Part model, mm, in its own coordinate system. Face numbers are marked on the shaded views. Round coordinates to 2 decimals unless told otherwise and drop trailing zeros. Loops run counter-clockwise (first coordinate to the right, second up) from the corner with the lowest first, then second, coordinate; pieces in that order, holes last. Notation, with made-up numbers: (39.5, -35.75) - (48.5, -35.75) arc R24 ccw to (48.5, -15.75) - close; hole circle Ø7 at (40, 37.5). An arc over 180 degrees is marked (long way). Write each question's results on one line, items separated by ' | '. Start each with the question number.
(1) Flat gauge pins, fed straight in: P1, Ø1, axis at x = 14, y = -1.5, coming from the -Z side; P2, Ø0.5, axis at y = 0, z = -62.5, coming from the -X side; P3, Ø2.5, axis at x = 7.5, y = -1.5, coming from the +Z side; P4, Ø3, axis at y = 0, z = 0, coming from the +X side. Where does each tip first touch, or does it go through?
(2) Cut at C-C, the plane z = -46.5. List the corners of the cut face in (x, y).
(3) Drill centre lines: L1, parallel to Y at x = 1, z = -106.5; L2, parallel to Y at x = 10.35, z = -117; L3, parallel to Z at x = -14, y = -0.75. Where is each one in solid material? Low to high.
(4) Cut at B-B, the plane z = 0. List the corners of the cut face in (x, y), then the cut area to 3 significant figures.
(5) Cut at A-A, the plane x = 0. Give the number of separate pieces and of enclosed holes in the cut face, then the cut area to 3 significant figures.
(6) Cut at D-D, the plane z = -13. List the corners of the cut face in (x, y), then the cut area to 3 significant figures.
(7) Mould opens along Z. For the marked faces 1, 2 and 3 say: released by +Z, released by -Z, zero draft, split by the parting line, or undercut.
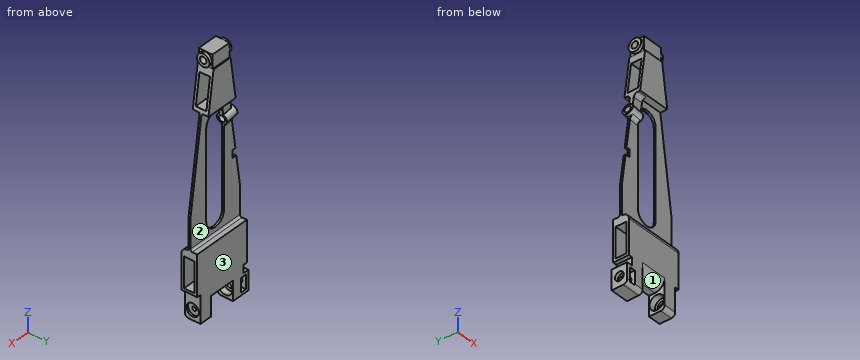
from build123d import *

# Parameters (mm, degrees)
JOINTTIBIA_DEPTH           = 3.5
JOINTTIBIA_DEPTH_BACK      = 3.5
ESQUISSE2_W                = 13.5
ESQUISSE2_H                = 7
ESQUISSE3_R                = 1.7
HOLEAXETIBIA_DEPTH         = 14.5
ESQUISSE4_R                = 5.505678288
ESQUISSE4_R_2              = 3.2
ENTRETOISETIBIA_DEPTH      = 1.5
SHAPEJOINTCOXA_DEPTH       = 4
SHAPEJOINTCOXA_DEPTH_BACK  = 4
ESQUISSE6_R                = 3.2
HOLEMAGNET_DEPTH           = 1
ESQUISSE7_R                = 2.25
HOLEAXE_DEPTH              = 8
ESQUISSE9_R                = 3.7
HOLEBEARING_DEPTH          = 3.2
ESQUISSE10_R               = 2.25
ENTRETOISEBEARING_DEPTH    = 1
ESQUISSE12_W               = 10
ESQUISSE12_H               = 8
ESQUISSE12_R               = 2.25
EXTSCREWLESS_DEPTH         = 3
ESQUISSE13_W               = 3
ESQUISSE13_H               = 7
SCEWLESSLOCKER_DEPTH       = 10
ESQUISSE24_W               = 30.5
ESQUISSE24_H               = 8
SHAPE_BDY_DEPTH            = 104.5
TRIANGULIZE_DEPTH          = 10
ESQUISSE27_W               = 15.4
ESQUISSE27_H               = 5.4
ATTACHWINGS_DEPTH          = 10
ESQUISSE29_W               = 62.63923601
ESQUISSE29_H               = 9.700813627
VOID_BODY_DEPTH            = 38
MASS_REMOVER_PCB_DEPTH     = 10
CONG_1_R                   = 5
CONG_2_R                   = 3
ESQUISSE32_W               = 15.4
ESQUISSE32_H               = 5.4
LOCKERHOLE_DEPTH           = 32
FIXATIONSENSOR_DEPTH       = 1.5
FIXATIONSENSOR_DEPTH_BACK  = 5
ESQUISSE33_R               = 2.6
ESQUISSE34_R               = 1.6
SCREWFIXATIONSENSOR_DEPTH  = 10
ESQUISSE35_W               = 8
ESQUISSE35_H               = 2
FIXATIONSENSORRENFOR_DEPTH = 5
CONG_3_R                   = 3
CONG_4_R                   = 2
CONG_5_R                   = 2
CONG_6_R                   = 1
ESQUISSE36_R               = 2
ENL_V_MAT_EXTRU_1_DEPTH    = 4.5
ESQUISSE38_R               = 1
REMOVER_HELPER_DEPTH       = 10


with BuildPart() as part:
    # Esquisse2 → JointTibia (new, two sides: drawn at the far end of the back side and taken through both)
    with BuildSketch(Plane(origin=(0, 0, 0), x_dir=(1, 0, 0), z_dir=(0, 1, 0)).offset(-JOINTTIBIA_DEPTH_BACK)):
        Rectangle(ESQUISSE2_W, ESQUISSE2_H)
    extrude(amount=JOINTTIBIA_DEPTH + JOINTTIBIA_DEPTH_BACK)

    # Esquisse3 → HoleAxeTibia (cut)
    with BuildSketch(Plane(origin=(6.75, 0, 0), x_dir=(0, 0, -1), z_dir=(1, 0, 0))):
        Circle(ESQUISSE3_R)
    extrude(amount=-HOLEAXETIBIA_DEPTH, mode=Mode.SUBTRACT)

    # Esquisse4 → EntretoiseTibia (cut)
    with BuildSketch(Plane(origin=(6.75, 0, 0), x_dir=(0, 0, -1), z_dir=(1, 0, 0))):
        Circle(ESQUISSE4_R)
        Circle(ESQUISSE4_R_2, mode=Mode.SUBTRACT)
    entretoisetibia = extrude(amount=-ENTRETOISETIBIA_DEPTH, mode=Mode.SUBTRACT)

    # Symétrie1: EntretoiseTibia across plane
    add(entretoisetibia.mirror(Plane(origin=(0, 0, 0), x_dir=(0, 0, 1), z_dir=(1, 0, 0))), mode=Mode.SUBTRACT)



with BuildPart() as body_2:
    # Esquisse5 → ShapeJointCoxa (new, two sides: drawn at the far end of the back side and taken through both)
    with BuildSketch(Plane(origin=(0, 0, 0), x_dir=(1, 0, 0), z_dir=(0, 1, 0)).offset(-SHAPEJOINTCOXA_DEPTH_BACK)):
        Polygon((-13.25, 112), (-13.25, 122), (-6.75, 122), (-6.75, 112), (6.75, 112), (6.75, 122), (13.25, 122), (13.25, 112), (13.25, 108), (-13.25, 108), align=None)
    extrude(amount=SHAPEJOINTCOXA_DEPTH + SHAPEJOINTCOXA_DEPTH_BACK)

    # Esquisse6 → HoleMagnet (cut)
    with BuildSketch(Plane(origin=(13.25, 0, 0), x_dir=(0, 0, -1), z_dir=(1, 0, 0))):
        with Locations((117, 0)):
            Circle(ESQUISSE6_R)
    extrude(amount=-HOLEMAGNET_DEPTH, mode=Mode.SUBTRACT)

    # Esquisse7 → HoleAxe (cut)
    with BuildSketch(Plane.ZY.offset(13.25)):
        with Locations((-117, 0)):
            Circle(ESQUISSE7_R)
    extrude(amount=-HOLEAXE_DEPTH, mode=Mode.SUBTRACT)

    # Esquisse9 → HoleBearing (cut)
    with BuildSketch(Plane.ZY.offset(-6.75)):
        with Locations((-117, 0)):
            Circle(ESQUISSE9_R)
    holebearing = extrude(amount=-HOLEBEARING_DEPTH, mode=Mode.SUBTRACT)

    # Symétrie2: HoleBearing across plane
    add(holebearing.mirror(Plane(origin=(0, 0, 0), x_dir=(0, 0, 1), z_dir=(1, 0, 0))), mode=Mode.SUBTRACT)

    # Esquisse10 → EntretoiseBearing (cut)
    with BuildSketch(Plane.ZY.offset(-9.95)):
        with Locations((-117, 0)):
            Circle(ESQUISSE10_R)
    extrude(amount=-ENTRETOISEBEARING_DEPTH, mode=Mode.SUBTRACT)

    # Esquisse12 → ExtScrewLess (add)
    with BuildSketch(Plane.ZY.offset(13.25)):
        with Locations((-117, 0)):
            Rectangle(ESQUISSE12_W, ESQUISSE12_H)
        with Locations((-117, 0)):
            Circle(ESQUISSE12_R, mode=Mode.SUBTRACT)
    extrude(amount=EXTSCREWLESS_DEPTH)

    # Esquisse13 → ScewLessLocker (cut)
    with BuildSketch(Plane(origin=(0, 4, 0), x_dir=(1, 0, 0), z_dir=(0, 1, 0))):
        with Locations((-13.1, 117)):
            Rectangle(ESQUISSE13_W, ESQUISSE13_H)
    extrude(amount=-SCEWLESSLOCKER_DEPTH, mode=Mode.SUBTRACT)


with BuildPart() as part_1:
    add(part.part)

    add(body_2.part)  # Shape_bdy merges body 2
    # Esquisse24 → Shape_bdy (add)
    with BuildSketch(Plane.XY.offset(-108)):
        Rectangle(ESQUISSE24_W, ESQUISSE24_H)
    extrude(amount=SHAPE_BDY_DEPTH)

    # Esquisse26 → Triangulize (cut)
    with BuildSketch(Plane.XZ.offset(4)):
        Polygon((-5.25, -3.5), (-15.25, -72), (-15.25, -3.5), align=None)
        Polygon((5.25, -3.5), (15.25, -3.5), (15.25, -72), align=None)
    extrude(amount=-TRIANGULIZE_DEPTH, mode=Mode.SUBTRACT)

    # Esquisse27 → AttachWings (cut)
    with BuildSketch(Plane(origin=(15.25, 0, 0), x_dir=(0, 0, -1), z_dir=(1, 0, 0))):
        with Locations((99, 0)):
            Rectangle(ESQUISSE27_W, ESQUISSE27_H)
        with Locations((15, 0)):
            Rectangle(ESQUISSE27_W, ESQUISSE27_H)
    attachwings = extrude(amount=-ATTACHWINGS_DEPTH, mode=Mode.SUBTRACT)

    # Symétrie4: AttachWings across plane
    add(attachwings.mirror(Plane(origin=(0, 0, 0), x_dir=(0, 0, 1), z_dir=(1, 0, 0))), mode=Mode.SUBTRACT)

    # Esquisse29 → Void body (cut)
    with BuildSketch(Plane(origin=(15.25, 0, 0), x_dir=(0, 0, -1), z_dir=(1, 0, 0))):
        with Locations((56.023105982, 5.350406814)):
            Rectangle(ESQUISSE29_W, ESQUISSE29_H)
        with Locations((56.023105982, -5.350406814)):
            Rectangle(ESQUISSE29_W, ESQUISSE29_H)
    extrude(amount=-VOID_BODY_DEPTH, mode=Mode.SUBTRACT)

    # Esquisse30 → Mass remover & PCB (cut)
    with BuildSketch(Plane(origin=(0, 0.5, 0), x_dir=(1, 0, 0), z_dir=(0, 1, 0))):
        with BuildLine():
            Line((5.5, 78.523105982), (5.5, 33.523105982))
            ThreePointArc((5.5, 33.523105982), (0, 28.023105982), (-5.5, 33.523105982))
            Line((-5.5, 33.523105982), (-5.5, 78.523105982))
            ThreePointArc((-5.5, 78.523105982), (0, 84.023105982), (5.5, 78.523105982))
        make_face()
    extrude(amount=-MASS_REMOVER_PCB_DEPTH, mode=Mode.SUBTRACT)

    # Congé1
    cong_1_edges = [part_1.edges().sort_by_distance(p)[0] for p in [
        (0, -4, -112),
    ]]
    fillet(cong_1_edges, radius=CONG_1_R)

    # Congé2
    cong_2_edges = [part_1.edges().sort_by_distance(p)[0] for p in [
        (0, -4, -87.342723987),
    ]]
    fillet(cong_2_edges, radius=CONG_2_R)

    # Esquisse32 → LockerHole (cut)
    with BuildSketch(Plane(origin=(5.25, 0, 0), x_dir=(0, 0, -1), z_dir=(1, 0, 0))):
        with Locations((99, 0)):
            Rectangle(ESQUISSE32_W, ESQUISSE32_H)
        with Locations((15, 0)):
            Rectangle(ESQUISSE32_W, ESQUISSE32_H)
    extrude(amount=-LOCKERHOLE_DEPTH, mode=Mode.SUBTRACT)

    # Esquisse33 → FixationSensor (add, two sides: drawn at the far end of the back side and taken through both)
    with BuildSketch(Plane(origin=(-4.640161198, 0, 0.677395795), x_dir=(0.14445423110427463, 0, 0.989511483064281), z_dir=(-0.989511483064281, 0, 0.14445423110427463)).offset(-FIXATIONSENSOR_DEPTH_BACK)):
        with Locations((-34.81506606, 0)):
            Circle(ESQUISSE33_R)
    extrude(amount=FIXATIONSENSOR_DEPTH + FIXATIONSENSOR_DEPTH_BACK)

    # Esquisse34 → ScrewFixationSensor (cut)
    with BuildSketch(Plane(origin=(-6.124428422, 0, 0.894077142), x_dir=(0.14445423110427466, 0, 0.989511483064281), z_dir=(-0.989511483064281, 0, 0.14445423110427466))):
        with Locations((-34.81506606, 0)):
            Circle(ESQUISSE34_R)
    extrude(amount=-SCREWFIXATIONSENSOR_DEPTH, mode=Mode.SUBTRACT)

    # Esquisse35 → FixationSensorRenfor (add)
    with BuildSketch(Plane(origin=(-4.640161198, 0, 0.677395795), x_dir=(0.14445423110427463, 0, 0.989511483064281), z_dir=(-0.989511483064281, 0, 0.14445423110427463))):
        with Locations((-28.41506606, 0)):
            Rectangle(ESQUISSE35_W, ESQUISSE35_H)
    extrude(amount=-FIXATIONSENSORRENFOR_DEPTH)

    # Congé3
    cong_3_edges = [part_1.edges().sort_by_distance(p)[0] for p in [
        (-7.768957729, 0.5, -36.628455586),
        (-7.768957729, -0.5, -36.628455586),
    ]]
    fillet(cong_3_edges, radius=CONG_3_R)

    # Congé4
    # the kernel refuses this fillet: 2 mm, written as the material it takes off along each edge
    with BuildSketch(Plane(origin=(1.75, -4, -122), x_dir=(0, 0, 1), z_dir=(1, 0, 0))) as cong_4_piece_1:
        with BuildLine():
            CenterArc((CONG_4_R, -CONG_4_R), CONG_4_R, 90, 90)
            Line((0, -CONG_4_R), (0, 0))
            Line((0, 0), (CONG_4_R, 0))
        make_face()
    extrude(amount=16.5, mode=Mode.SUBTRACT)
    with BuildSketch(Plane(origin=(-21.25, -4, -122), x_dir=(0, 0, 1), z_dir=(1, 0, 0))) as cong_4_piece_2:
        with BuildLine():
            CenterArc((CONG_4_R, -CONG_4_R), CONG_4_R, 90, 90)
            Line((0, -CONG_4_R), (0, 0))
            Line((0, 0), (CONG_4_R, 0))
        make_face()
    extrude(amount=19.5, mode=Mode.SUBTRACT)

    # Congé5
    cong_5_edges = [part_1.edges().sort_by_distance(p)[0] for p in [
        (-5.818900475, 1, -24.703487977),
        (-5.818900475, -1, -24.703487977),
    ]]
    fillet(cong_5_edges, radius=CONG_5_R)

    # Congé6
    cong_6_edges = [part_1.edges().sort_by_distance(p)[0] for p in [
        (0, 0.5, -87.342723987),
        (2.52649923, 0.5, -24.703487977),
    ]]
    fillet(cong_6_edges, radius=CONG_6_R)

    # Esquisse36 → Enlèv. mat.-Extru.1 (cut)
    with BuildSketch(Plane.ZY.offset(15.25)):
        with Locations((-54.7, 0)):
            Circle(ESQUISSE36_R)
    extrude(amount=-ENL_V_MAT_EXTRU_1_DEPTH, mode=Mode.SUBTRACT)

    # Esquisse38 → Remover helper (cut)
    with BuildSketch(Plane(origin=(12.25, 0, 0), x_dir=(0, 0, -1), z_dir=(1, 0, 0))):
        with Locations((117, 0)):
            Circle(ESQUISSE38_R)
    extrude(amount=-REMOVER_HELPER_DEPTH, mode=Mode.SUBTRACT)


solid = part_1.part
A:
1) P1: z = -108 | P2: x = -13.9 | P3: z = 3.16 | P4: through
2) outline: (-11.53, -0.5) - (-5.5, -0.5) - (-5.5, 0.5) - (-11.53, 0.5) - close; (5.5, -0.5) - (11.53, -0.5) - (11.53, 0.5) - (5.5, 0.5) - close
3) L1: -4 to -2.7, 2.7 to 4 | L2: -4 to -2.25, 2.25 to 4 | L3: -122 to -120.5, -113.5 to -112, -108 to -106.7, -91.3 to -87.34
4) outline: (-6.75, -3.2) - (-5.25, -3.2) - (-5.25, -3.5) - (5.25, -3.5) - (5.25, -3.2) - (6.75, -3.2) - (6.75, -1.7) - (-6.75, -1.7) - close; (-6.75, 1.7) - (6.75, 1.7) - (6.75, 3.2) - (5.25, 3.2) - (5.25, 3.5) - (-5.25, 3.5) - (-5.25, 3.2) - (-6.75, 3.2) - close | area: 46.8 mm2
5) separate pieces: 2 | enclosed holes: 3 | area: 240 mm2
6) outline: (-6.64, -4) - (6.64, -4) - (6.64, -2.7) - (-6.64, -2.7) - close; (-6.64, 2.7) - (6.64, 2.7) - (6.64, 4) - (-6.64, 4) - close | area: 34.5 mm2
7) face 1: released by -Z | face 2: undercut | face 3: zero draft
